Part model, mm, in its own coordinate system. Face numbers are marked on the shaded views. A direction names the side the tool comes from. Round coordinates to 2 decimals unless told otherwise and drop trailing zeros. Order: outer loops, then holes, each group sorted by start corner. A loop starts at its lowest first (then second) coordinate and runs counter-clockwise, first axis right, second up. Notation, with made-up numbers: (19, 68.25) - (39, 68.25) arc R8 cw to (39, 74.25) - close; hole circle Ø6 at (74.5, 37.25). An arc over 180 degrees is marked (long way). Answer as a JSON object with one key per item and string values.
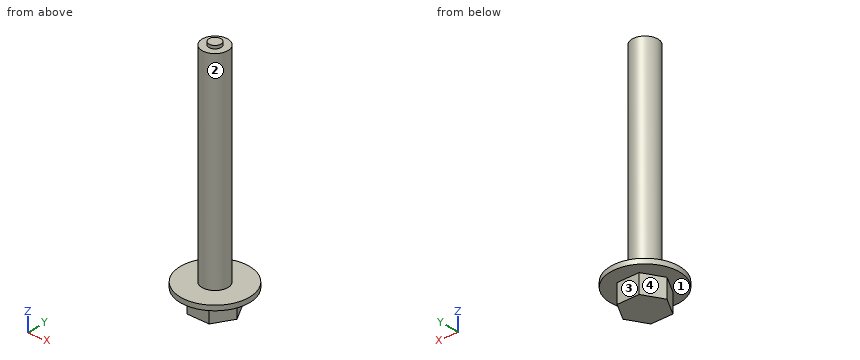
```python
from build123d import *

# Parameters (mm, degrees)
BOSS_EXTRUDE1_DEPTH     = 3.175
SKETCH2_R               = 5.715
BOSS_EXTRUDE2_DEPTH     = 0.8128
CUT_EXTRUDE1_DEPTH      = 51.094096647
CUT_EXTRUDE1_DEPTH_BACK = 51.094096647
SKETCH4_W               = 11.07
SKETCH4_H               = 6


with BuildPart() as part:
    # Sketch1 → Boss-Extrude1 (new body)
    with BuildSketch(Plane.XY):
        Polygon((3.666174209, 0), (1.833087105, 3.175), (-1.833087105, 3.175), (-3.666174209, 0), (-1.833087105, -3.175), (1.833087105, -3.175), align=None)
    extrude(amount=BOSS_EXTRUDE1_DEPTH)

    # Sketch2 → Boss-Extrude2 (add)
    with BuildSketch(Plane.XY.offset(3.175)):
        Circle(SKETCH2_R)
    extrude(amount=BOSS_EXTRUDE2_DEPTH)

    # Sketch3 → Revolve1 (revolve)
    with BuildSketch(Plane(origin=(0, 0, 0), x_dir=(0, 0, -1), z_dir=(1, 0, 0)), mode=Mode.PRIVATE) as revolve1_sk:
        Polygon((-3.9878, 0), (-49.4378, 0), (-49.4378, 2.145), (-39.3678, 2.145), (-39.3678, 1), (-38.3678, 1), (-38.3678, 2.145), (-3.9878, 2.145), align=None)
    revolve(revolve1_sk.sketch.rotate(Axis((0, 0, 3.9878), (0, 0, 1)), 90), axis=Axis((0, 0, 3.9878), (0, 0, 1)))

    # Sketch4 → Cut-Extrude1 (cut, two sides: drawn at the far end of the back side and taken through both)
    with BuildSketch(Plane(origin=(0, 0, 0), x_dir=(0, 0, -1), z_dir=(1, 0, 0)).offset(-CUT_EXTRUDE1_DEPTH_BACK)):
        with Locations((-44.4028, 0)):
            Rectangle(SKETCH4_W, SKETCH4_H)
    extrude(amount=CUT_EXTRUDE1_DEPTH + CUT_EXTRUDE1_DEPTH_BACK, mode=Mode.SUBTRACT)


solid = part.part
```
Item 1: Cut at A-A (x = 0). Write the cut outline in (y, z) (3 decimals).
Taken from the geometry:
{"outline": "(-5.715, 3.175) - (-3.175, 3.175) - (-3.175, 0) - (3.175, 0) - (3.175, 3.175) - (5.715, 3.175) - (5.715, 3.988) - (2.145, 3.988) - (2.145, 38.368) - (1, 38.368) - (1, 38.868) - (-1, 38.868) - (-1, 38.368) - (-2.145, 38.368) - (-2.145, 3.988) - (-5.715, 3.988) - close"}
Item 2: Drop flat-ended pins along their axis: P1, Ø2, axis at x = -0.5, z = 29.5, coming from the -Y side (3 decimals); P2, Ø3.5, axis at x = 2.5, y = 2, coming from the +Z side; P3, Ø1.5, axis at x = -3.5, y = -4.5, coming from the +Z side. Give the stop position or say it passes through.
Taken from the geometry:
{"P1": "y = -2.145", "P2": "z = 38.37", "P3": "z = 3.99"}
Item 3: Cut at C-C (z = 16.5). Write the cut outline in (x, y) (3 decimals), plus the area to 3 significant figures.
Taken from the geometry:
{"outline": "circle Ø4.29 at (0, 0)", "area": "14.5 mm2"}
Item 4: Cut at D-D (x = -2.5). Write the cut outline in (y, z) (3 decimals).
Taken from the geometry:
{"outline": "(-5.139, 3.175) - (-2.02, 3.175) - (-2.02, 0) - (2.02, 0) - (2.02, 3.175) - (5.139, 3.175) - (5.139, 3.988) - (-5.139, 3.988) - close"}
Item 5: Tool access for the marked faces 1, 2, 3 and 4: list every direction of +Z, -Z, +X, -X, +Y, -Y with a clear straight run to the whole face (end or side of a thin tool).
Taken from the geometry:
{"face 1": "-Z", "face 2": "+Z", "face 3": "-Z, +X, -X, +Y", "face 4": "-Z, -X, +Y"}
Item 6: Probe L1, parallel to Z at x = 3, y = -4.5 (3 decimals); L2, parallel to Z at x = 0.5, y = -2.5; L3, parallel to Y at x = 0, z = 3 (3 decimals). List the from-to ranges inside material, lowest first. Write a range as from..to.
Taken from the geometry:
{"L1": "3.175..3.988", "L2": "0..3.99", "L3": "-3.175..3.175"}
Item 7: Cut at B-B (y = 2.5). Write the cut outline in (x, z) (3 decimals).
Taken from the geometry:
{"outline": "(-5.139, 3.175) - (-2.223, 3.175) - (-2.223, 0) - (2.223, 0) - (2.223, 3.175) - (5.139, 3.175) - (5.139, 3.988) - (-5.139, 3.988) - close"}
